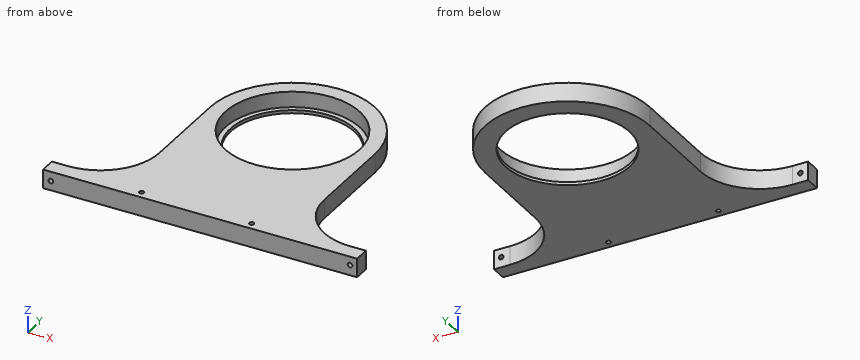
Autodesk Fusion 360 part; units mm, degrees
sketch "Sketch1" plane through (0, 0, 0) normal (0, 0, 1) x (1, 0, 0)
  circle A0 centre (0, 0) radius 42.75
  circle A1 centre (0, 0) radius 39.5
  line L0 (0, 0) -> (0, -100) construction
  line L1 (100, -105) -> (-100, -105)
  line L2 (-100, -105) -> (-100, -95)
  line L3 (100, -95) -> (100, -105)
  line L4 (100, -105) -> (-100, -95) construction
  line L5 (-100, -105) -> (100, -95) construction
  circle A2 centre (0, 0) radius 52.5
  line L6 (-52.5, 0) -> (-52.5, -57.5)
  line L7 (52.5, 0) -> (52.5, -57.5)
  line L8 (-100, -95) -> (-90, -95)
  line L9 (90, -95) -> (100, -95)
  arc A3 (-90, -95) -> (-52.5, -57.5) centre (-90, -57.5) ccw
  arc A4 (52.5, -57.5) -> (90, -95) centre (90, -57.5) ccw
  line L10 (100, -100) -> (30, -100) construction
  line L11 (100, -100) -> (-40, -100) construction
  circle A5 centre (30, -100) radius 1.5
  circle A6 centre (-40, -100) radius 1.5
  point P0 (0, -100)
  dimension "d1" = 85.5
  dimension "d5" = 79
  dimension "d7" = 100
  dimension "d8" = 200
  dimension "d9" = 10
  dimension "d10" = 105
  dimension "d11" = 37.5
  dimension "d12" = 10
  dimension "d13" = 37.5
  dimension "d24" = 70
  dimension "d25" = 140
  dimension "d26" = 3
  dimension "d27" = 3
extrude "Extrude1" add sketch "Sketch1" along normal blind 12 contours L1 L2 L3 A2 L6 L7 L8 L9 A3 A4 | A2
extrude "Extrude2" add sketch "Sketch1" along normal blind 2 contours A0
hole "Hole1" at (-95, -95, 6) direction (0, -1, 0) diameter 3 depth 10 tip angle 118
hole "Hole2" at (95.5037, -95, 6.5484) direction (0, -1, 0) diameter 3 depth 10 tip angle 118
equation "d1 = BearingDia + Tollerance"
equation "BearingDia = 85 mm"
equation "BearingOffset = 79 mm"
equation "Tollerance = 0.5 mm"
equation "d5 = BearingOffset"
equation "AxleHeight = 105 mm"
equation "d7 = AxleHeight - 5 mm"
equation "d10 = BearingDia + 20 mm"
equation "d24 = ( 210 / 3 ) * 1 mm"
Geometry check sheet. Reference: the model listing, model coordinates, mm. Coordinates: 2 decimals unless noted, no trailing zeros. Order: outer loops, then holes, each group sorted by start corner. A loop starts at its lowest first (then second) coordinate and runs counter-clockwise, first axis right, second up.
Item 1: Section check D-D (y = -60.5). Enter the section's corners in (x, z).
Item 2: Scan lines: line 1 along X through (y, z) = (-100, 4); line 2 along Y through (x, z) = (30, 7.5); line 3 along X through (y, z) = (-100.75, 6). Record each from-to range of solid material in increasing order.
Item 3: Depth check by flat-ended pin: pin 1 (2 mm diameter, centred on x = -62.5, z = 3.5, fed in from +Y); pin 2 (4 mm diameter, centred on x = -95, z = 6, fed in from +Y); pin 3 (6 mm diameter, centred on y = -18, z = 6, fed in from -X); pin 4 (2.5 mm diameter, centred on x = -40, y = -100, fed in from -Z). Enter the tip coordinate at first touch or a pass-through.
Item 4: Section check C-C (x = -55.5). Enter the section's corners in (y, z), plus the area to 3 significant figures.
Item 5: Section check A-A (y = -6). Enter the section's corners in (x, z), plus the area to 3 significant figures.
Item 6: Section check B-B (x = 0). Enter the section's corners in (y, z).
Check sheet entries:
1. outline: (-52.62, 0) - (52.62, 0) - (52.62, 12) - (-52.62, 12) - close
2. line 1: x = -100 to -41.5, -38.5 to 28.5, 31.5 to 100
2. line 2: y = -105 to -101.5, -98.5 to -30.46, 30.46 to 43.08
2. line 3: x = -100 to -96.5, -93.5 to -41.3, -38.7 to 28.7, 31.3 to 94.11, 96.9 to 100
3. pin 1: stops at y = -81.87
3. pin 2: stops at y = -95
3. pin 3: stops at x = -52.5
3. pin 4: passes through
4. outline: (-105, 0) - (-72.2, 0) - (-72.2, 12) - (-105, 12) - close
4. area: 394 mm2
5. outline: (-52.5, 0) - (-39.04, 0) - (-39.04, 2) - (-42.33, 2) - (-42.33, 12) - (-52.5, 12) - close; (39.04, 0) - (52.5, 0) - (52.5, 12) - (42.33, 12) - (42.33, 2) - (39.04, 2) - close
5. area: 257 mm2
6. outline: (-105, 0) - (-39.5, 0) - (-39.5, 2) - (-42.75, 2) - (-42.75, 12) - (-105, 12) - close; (39.5, 0) - (52.5, 0) - (52.5, 12) - (42.75, 12) - (42.75, 2) - (39.5, 2) - close
